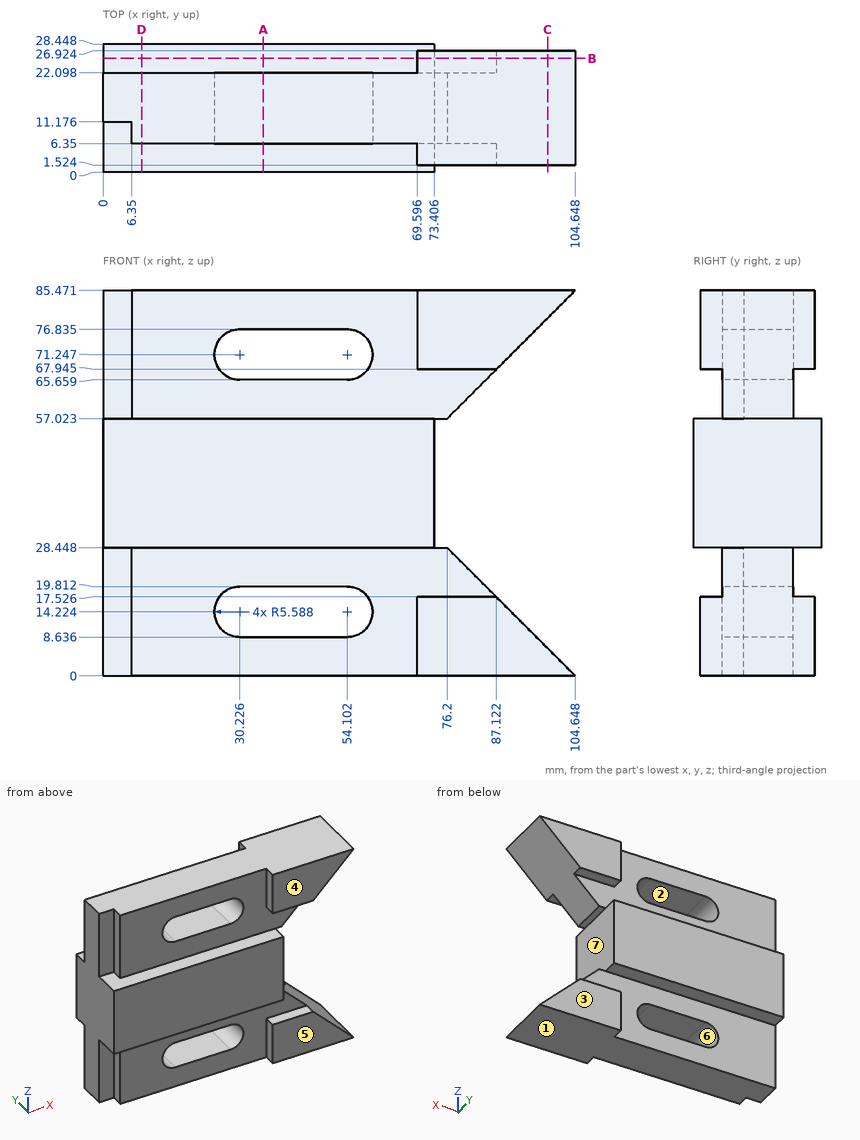
The drawing under review shows one solid part. Ordinate dimensions are in mm from its lowest x, y, z. A direction names the side the tool comes from. Coordinates: 2 decimals unless noted, no trailing zeros. Loops run counter-clockwise (first coordinate to the right, second up) from the corner with the lowest first, then second, coordinate; pieces in that order, holes last.
Item 1: Wall thickness on L1, parallel to Z at x = 48, y = 7.5 (3 decimals); L2, parallel to Z at x = 72, y = 5.25 (3 decimals); L3, parallel to X at y = 17.5, z = 47: over which ranges is each line inside the solid? List them lowest first.
Completed:
L1: z = 0 to 8.636, 19.812 to 65.659, 76.835 to 85.471
L2: z = 0 to 17.526, 28.448 to 57.023, 67.945 to 85.471
L3: x = 0 to 73.41
Item 2: Add section B-B (y = 25.25). Write out the cut boundary in (x, z) (3 decimals), and give its area (3 significant figures).
Completed:
outline: (0, 28.448) - (73.406, 28.448) - (73.406, 57.023) - (0, 57.023) - close; (69.596, 0) - (104.648, 0) - (87.122, 17.526) - (69.596, 17.526) - close; (69.596, 67.945) - (87.122, 67.945) - (104.648, 85.471) - (69.596, 85.471) - close
area: 3,020 mm2
Item 3: Draft analysis for pull direction Z (two halves, no side actions). For the marked faces 1, 2 and 3, state which applies: pulls with the +Z half, pulls with the -Z half, needs draft (parallel to the pull), parting line crosses it, or undercut.
Completed:
face 1: pulls with the -Z half
face 2: undercut
face 3: needs draft
Item 4: Add section C-C (x = 98.5). Write out the cut boundary in (y, z), and give its area (3 significant figures).
Completed:
outline: (1.52, 0) - (26.92, 0) - (26.92, 6.15) - (1.52, 6.15) - close; (1.52, 79.32) - (26.92, 79.32) - (26.92, 85.47) - (1.52, 85.47) - close
area: 312 mm2
Item 5: Add section A-A (x = 35.5). Write out the cut boundary in (y, z) (3 decimals).
Completed:
outline: (0, 28.448) - (6.35, 28.448) - (6.35, 19.812) - (22.098, 19.812) - (22.098, 28.448) - (28.448, 28.448) - (28.448, 57.023) - (22.098, 57.023) - (22.098, 65.659) - (6.35, 65.659) - (6.35, 57.023) - (0, 57.023) - close; (6.35, 0) - (22.098, 0) - (22.098, 8.636) - (6.35, 8.636) - close; (6.35, 76.835) - (22.098, 76.835) - (22.098, 85.471) - (6.35, 85.471) - close
Item 6: Clearance check with flat-ended pins moving along their axes: pin 1 (1.5 mm diameter, centred on y = 16.5, z = 22.5, fed in from +X); pin 2 (1.4 mm diameter, centred on y = 4, z = 76.5, fed in from -X); pin 3 (19.5 mm diameter, centred on x = 87.5, z = 7, fed in from +Y). State where each tip first meets the part, or that it passes through.
Completed:
pin 1: stops at x = 82.9
pin 2: stops at x = 69.6
pin 3: stops at y = 26.92
Item 7: For the marked faces 4, 5, 6 and 7, list the 3-axis set-ups (+Z, -Z, +X, -X, +Y, -Y) from which the entire face can be reached by the end or side of a thin tool; tool diameter is ignored.
Completed:
face 4: +Z, +X, -X, -Y
face 5: -Z, +X, -X, -Y
face 6: +Y, -Y
face 7: +X, +Y, -Y
Item 8: Add section D-D (x = 8.5). Write out the cut boundary in (y, z).
Completed:
outline: (0, 28.45) - (6.35, 28.45) - (6.35, 0) - (22.1, 0) - (22.1, 28.45) - (28.45, 28.45) - (28.45, 57.02) - (22.1, 57.02) - (22.1, 85.47) - (6.35, 85.47) - (6.35, 57.02) - (0, 57.02) - close
